```python
from build123d import *

# Parameters (mm, degrees)
F0_R     = 1.5875
F1_DEPTH = 10.16
F2_DEPTH = 38.1
F3_W     = 10.16
F3_H     = 10.16
F3_W_2   = 25.4
F3_H_2   = 50.8
F4_DEPTH = 5.08
F5_DEPTH = 3.81
F6_R     = 5.07999


# Not quite as in the source:
# - a fillet or chamfer is up to 0.001 mm smaller than in the source, because OpenCascade refuses the exact size
# - a feature names something its author has since deleted; it is built from what else it names


with BuildPart() as f1:
    # F0 (on Top) → F1 (new body)
    with BuildSketch(Plane.XY):
        Polygon((24.5562880617, 49.3353436351), (14.3962880617, 49.3353436351), (14.3962880617, -7.8146563649), (14.3962880617, -39.5646563649), (14.3962880617, -64.9646563649), (24.5562880617, -64.9646563649), align=None)
        with Locations((19.4762880617, -39.5646563649)):
            Circle(F0_R, mode=Mode.SUBTRACT)
        with Locations((19.4762880617, -52.2646563649)):
            Circle(F0_R, mode=Mode.SUBTRACT)
    extrude(amount=F1_DEPTH)

    # F0 (on Top) → F2 (join)
    with BuildSketch(Plane.XY):
        with Locations((19.4762880617, -39.5646563649)):
            Circle(F0_R)
        with Locations((19.4762880617, -52.2646563649)):
            Circle(F0_R)
    extrude(amount=F2_DEPTH)

    # F3 (on face) → F4 (join)
    with BuildSketch(Plane(origin=(0, 49.3353436351, 0), x_dir=(-1, 0, 0), z_dir=(0, 1, 0))):
        with BuildLine():
            Line((-24.5562880617, 0), (-24.5562880617, 10.16))
            Line((-24.5562880617, 10.16), (-24.5562880617, 15.24))
            Line((-24.5562880617, 15.24), (-37.2562880617, 15.24))
            Line((-37.2562880617, 15.24), (-37.2562880617, -35.56))
            Line((-37.2562880617, -35.56), (-30.9062880617, -29.15440273))
            ThreePointArc((-30.9062880617, -29.15440273), (-19.3773342754, -21.5585615124), (-7.7287880617, -28.9696984238))
            Line((-7.7287880617, -28.9696984238), (-1.6962880617, -35.56))
            Line((-1.6962880617, -35.56), (-1.6962880617, 10.16))
            Line((-1.6962880617, 10.16), (-14.3962880617, 10.16))
            Line((-14.3962880617, 10.16), (-14.3962880617, 0))
            Line((-14.3962880617, 0), (-24.5562880617, 0))
        make_face()
        Polygon((-24.5562880617, 15.24), (-24.5562880617, 10.16), (-14.3962880617, 10.16), (-1.6962880617, 10.16), (-1.6962880617, 15.24), (-13.7612880617, 15.24), align=None)
        with Locations((-19.4762880617, 5.08)):
            Rectangle(F3_W, F3_H)
        with Locations((-49.9562880617, -10.16)):
            Rectangle(F3_W_2, F3_H_2)
        Polygon((-1.6962880617, 15.24), (-1.6962880617, 10.16), (-1.6962880617, -35.56), (23.7037119383, -35.56), (23.7037119383, 15.24), align=None)
    extrude(amount=F4_DEPTH)

    # F3 (on face) → F5 (join)
    with BuildSketch(Plane(origin=(0, 49.3353436351, 0), x_dir=(-1, 0, 0), z_dir=(0, 1, 0))):
        with Locations((-19.4762880617, 5.08)):
            Rectangle(F3_W, F3_H)
    extrude(amount=F5_DEPTH)

    # F6 (radius 5.08 in the source; OpenCascade refuses exactly that, so slightly less here)
    f6_edges = [f1.edges().sort_by_distance(p)[0] for p in [
        (19.377334, 54.415344, -21.558562),
        (4.712538, 54.415344, -32.264849),
        (34.081288, 54.415344, -32.357201),
    ]]
    fillet(f6_edges, radius=F6_R)


solid = f1.part
```
The model under review builds one solid part; all positions refer to its coordinate system, in mm. A direction names the side the tool comes from. Coordinates: 2 decimals unless noted, no trailing zeros. Write each loop counter-clockwise with the first axis right and the second up, starting at its lowest first coordinate (ties: lowest second). Pieces come first, ordered by that corner, then holes. Notation, with made-up numbers: (42, -1) - (83, -1) arc R14 cw to (83, 6) - close; hole circle Ø5 at (20.25, 71). An arc over 180 degrees is marked (long way). Answer in a Markdown table with one row per item. Add a question column.
Q1. To check wall thickness, follow line 1 along Y through (x, z) = (-1.5, 5); line 2 along Z through (x, y) = (21, 8.5); line 3 along X through (y, z) = (8, 3). State the ranges of each line that lie inside material, in increasing order. Write a range as from..to.
Q2. Clearance check with flat-ended pins moving along their axes: pin 1 (4 mm diameter, centred on y = -37.5, z = 11.5, fed in from +X); pin 2 (2.5 mm diameter, centred on x = 39.5, y = 53, fed in from +Z); pin 3 (5 mm diameter, centred on y = -33, z = 3.5, fed in from -X). State where each tip first meets the part, or that it passes through.
Q3. Consider section C-C on z = 26.5. Give the boundary of the cut face in (x, y) (1 decimal), then the cut area to 3 significant figures.
Q4. Consider section A-A on z = 3. Give the boundary of the cut face in (x, y).
Q5. Draft analysis for pull direction X (two halves, no side actions). For faces 4 (the face through (2.971, 52.967, -31.905)), 5 (the face through (14.396, -7, 5)), 6 (the face through (19, -40, 38.1)), 7 (the face through (19.27, -50.69, 23.93)), state which applies: +X half, -X half, draft (parallel to the pull), parting line (faces both ways), or undercut.
Q6. Consider section B-B on y = -19. Give the boundary of the cut face in (x, z).
Q7. For faces 1 (the face through (19.132, -41.114, 23.934)), 2 (the face through (24.556, -9, 5)), 3 (the face through (19, -7, 0)), list the 3-axis set-ups (+Z, -Z, +X, -X, +Y, -Y) from which the entire face can be reached by the end or side of a thin tool; tool diameter is ignored.
Q8. Consider section D-D on x = 51. Give the boundary of the cut face in (y, z), then the cut area to 3 significant figures.
Answers below:
| question | item | result |
|---|---|---|
| 1 | line 1 | 49.34..54.42 |
| 1 | line 2 | 0..10.16 |
| 1 | line 3 | 14.4..24.56 |
| 2 | pin 1 | x = 24.56 |
| 2 | pin 2 | z = 15.24 |
| 2 | pin 3 | x = 14.4 |
| 3 | outline | circle Ø3.2 at (19.5, -52.3); circle Ø3.2 at (19.5, -39.6) |
| 3 | area | 15.8 mm² |
| 4 | outline | (-23.7, 49.34) - (14.4, 49.34) - (14.4, -64.96) - (24.56, -64.96) - (24.56, 49.34) - (62.66, 49.34) - (62.66, 54.42) - (-23.7, 54.42) - close |
| 5 | face 4 | undercut |
| 5 | face 5 | -X half |
| 5 | face 6 | draft |
| 5 | face 7 | parting line |
| 6 | outline | (14.4, 0) - (24.56, 0) - (24.56, 10.16) - (14.4, 10.16) - close |
| 7 | face 1 | +Z |
| 7 | face 2 | +Z, -Z, +X, -Y |
| 7 | face 3 | -Z, +X, -X, -Y |
| 8 | outline | (49.34, -35.56) - (54.42, -35.56) - (54.42, 15.24) - (49.34, 15.24) - close |
| 8 | area | 258 mm² |
